```python
from build123d import *

# Parameters (mm, degrees)
PAD_DEPTH       = 5
POCKET_DEPTH    = 3
SKETCH002_R     = 5
SKETCH002_R_2   = 2
PAD001_DEPTH    = 14
FILLET_R        = 1
FILLET001_R     = 1
FILLET002_R     = 1
FILLET003_R     = 1
SKETCH003_R     = 10
POCKET001_DEPTH = 5.001
SKETCH004_R     = 2
POCKET002_DEPTH = 5.001
FILLET004_R     = 1
FILLET005_R     = 1
FILLET006_R     = 2
FILLET007_R     = 2


with BuildPart() as part:
    # Sketch → Pad (new body)
    with BuildSketch(Plane.XY):
        Polygon((0, 39), (-39, 0), (0, -39), (39, 0), align=None)
    extrude(amount=PAD_DEPTH)

    # Sketch001 → Pocket (cut)
    with BuildSketch(Plane.XY.offset(5)):
        Polygon((-42.5, 2.5), (-2.5, 2.5), (-2.5, 42.5), (2.5, 42.5), (2.5, 2.5), (42.5, 2.5), (42.5, -2.5), (2.5, -2.5), (2.5, -42.5), (-2.5, -42.5), (-2.5, -2.5), (-42.5, -2.5), align=None)
    extrude(amount=-POCKET_DEPTH, mode=Mode.SUBTRACT)

    # Sketch002 → Pad001 (new body)
    with BuildSketch(Plane.XY.offset(5)):
        with Locations((10.606602, 10.606602)):
            Circle(SKETCH002_R)
        with Locations((10.606602, 10.606602)):
            Circle(SKETCH002_R_2, mode=Mode.SUBTRACT)
        with Locations((-10.606602, -10.606602)):
            Circle(SKETCH002_R)
        with Locations((-10.606602, -10.606602)):
            Circle(SKETCH002_R_2, mode=Mode.SUBTRACT)
    extrude(amount=PAD001_DEPTH)

    # Fillet
    fillet_edges = [part.edges().sort_by_distance(p)[0] for p in [
        (-39, 0, 1),
    ]]
    fillet(fillet_edges, radius=FILLET_R)

    # Fillet001
    fillet001_edges = [part.edges().sort_by_distance(p)[0] for p in [
        (0, -39, 1),
    ]]
    fillet(fillet001_edges, radius=FILLET001_R)

    # Fillet002
    fillet002_edges = [part.edges().sort_by_distance(p)[0] for p in [
        (39, 0, 1),
    ]]
    fillet(fillet002_edges, radius=FILLET002_R)

    # Fillet003
    fillet003_edges = [part.edges().sort_by_distance(p)[0] for p in [
        (0, 39, 1),
    ]]
    fillet(fillet003_edges, radius=FILLET003_R)

    # Sketch003 → Pocket001 (cut, through all)
    with BuildSketch(Plane.XY.offset(5)):
        Circle(SKETCH003_R)
    extrude(amount=-POCKET001_DEPTH, mode=Mode.SUBTRACT)

    # Sketch004 → Pocket002 (cut, through all)
    with BuildSketch(Plane.XY.offset(5)):
        with Locations((-10.606602, -10.606602)):
            Circle(SKETCH004_R)
        with Locations((10.606602, 10.606602)):
            Circle(SKETCH004_R)
    extrude(amount=-POCKET002_DEPTH, mode=Mode.SUBTRACT)

    # Fillet004
    fillet004_edges = [part.edges().sort_by_distance(p)[0] for p in [
        (-7.071068, 7.071068, 5),
    ]]
    fillet(fillet004_edges, radius=FILLET004_R)

    # Fillet005
    fillet005_edges = [part.edges().sort_by_distance(p)[0] for p in [
        (7.071068, -7.071068, 5),
    ]]
    fillet(fillet005_edges, radius=FILLET005_R)

    # Fillet006
    fillet006_edges = [part.edges().sort_by_distance(p)[0] for p in [
        (5.606602, 10.606602, 19),
    ]]
    fillet(fillet006_edges, radius=FILLET006_R)

    # Fillet007
    fillet007_edges = [part.edges().sort_by_distance(p)[0] for p in [
        (-15.606602, -10.606602, 19),
    ]]
    fillet(fillet007_edges, radius=FILLET007_R)


solid = part.part
```
The listing builds one solid part. Answer for the finished solid, in the listing's coordinates (mm). A direction names the side the tool comes from. Coordinates: 2 decimals unless noted, no trailing zeros. Write each loop counter-clockwise with the first axis right and the second up, starting at its lowest first coordinate (ties: lowest second). Pieces come first, ordered by that corner, then holes. Notation, with made-up numbers: (33, -26.5) - (84, -26.5) arc R6 cw to (84, -22.5) - close; hole circle Ø2 at (56.25, 13.5). An arc over 180 degrees is marked (long way). Return JSON: item names as keys, results as strings. Group by question number.
1. Which of the six approach directions +Z, -Z, +X, -X, +Y, -Y give full straight-line access (tool end or side, diameter ignored) to faces 4 (the flat face through (-24, 0, 2)), 5 (the cylindrical face through (9.523, 5.726, 10.916)), 6 (the flat face through (0, 24, 2))?
2. Given pin 1 (3 mm diameter, centred on x = -9.5, y = 2, fed in from +Z); pin 2 (2.5 mm diameter, centred on y = -18.5, z = 3.5, fed in from -X); pin 3 (1.5 mm diameter, centred on y = 19.5, z = 3, fed in from +X), each flat-ended and moving along its own axis, determine where each tip first touches the part or whether it passes through.
3. A cutting plane is placed at C-C, the plane z = 6.5. Determine the outline of the cut face in (x, y), plus the area to 3 significant figures.
4. Determine the mould class of faces 1 (the flat face through (23, 2.5, 4)), 2 (the flat face through (19, -20, 2)), 3 (the cylindrical face through (-14.574, -13.649, 10.916)) for opening direction Y: released by +Y, released by -Y, zero draft, split by the parting line, or undercut.
5. A cutting plane is placed at A-A, the plane x = 24. Determine the outline of the cut face in (y, z).
6. Straight lines are drawn through the part: L1, parallel to X at y = 0, z = 1.35; L2, parallel to Y at x = -11.5, z = 4. For each, find the intervals that lie inside material, in ascending order.
7. A cutting plane is placed at B-B, the plane y = 31.5. Determine the outline of the cut face in (x, z).
Ans:
{
 "1": {"face 4": "+Z, +X, -X", "face 5": "+Z", "face 6": "+Z, +Y, -Y"},
 "2": {"pin 1": "z = 5", "pin 2": "x = -21.75", "pin 3": "x = 20.25"},
 "3": {"outline": "circle Ø10 at (-10.61, -10.61); circle Ø10 at (10.61, 10.61); hole circle Ø4 at (-10.61, -10.61); hole circle Ø4 at (10.61, 10.61)", "area": "132 mm²"},
 "4": {"face 1": "undercut", "face 2": "released by -Y", "face 3": "split by the parting line"},
 "5": {"outline": "(-15, 0) - (15, 0) - (15, 5) - (2.5, 5) - (2.5, 2) - (-2.5, 2) - (-2.5, 5) - (-15, 5) - close"},
 "6": {"L1": "-38.59 to -10, 10 to 38.59", "L2": "-27.5 to -12.4, -8.82 to -2.5, 2.5 to 27.5"},
 "7": {"outline": "(-7.5, 0) - (7.5, 0) - (7.5, 5) - (2.5, 5) - (2.5, 2) - (-2.5, 2) - (-2.5, 5) - (-7.5, 5) - close"}
}
